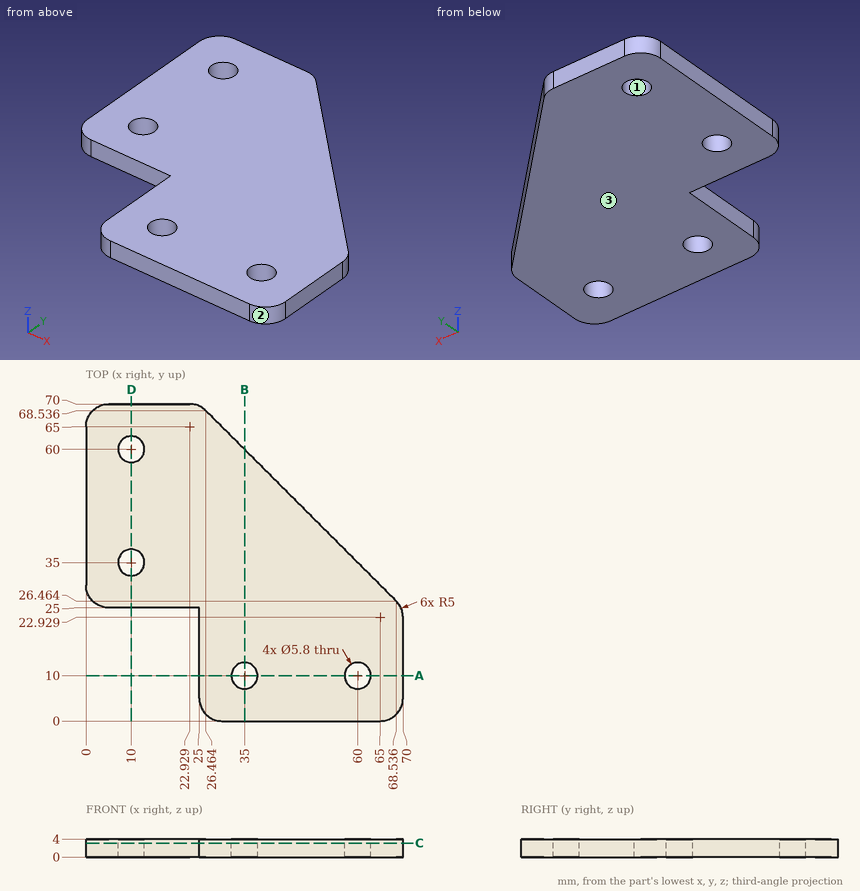
Answer from the drawing. Dimensions are ordinates in mm from the lowest x, y and z of the part. Give positions to 0.01 mm unless a question says otherwise; leave off trailing zeros. Loops run counter-clockwise (first coordinate to the right, second up) from the corner with the lowest first, then second, coordinate; pieces in that order, holes last. Notation, with made-up numbers: M -29.5,28.25 L 26.5,28.25 A7 ccw 26.5,36.25 Z; hole C 28,51.5 d7. An arc over 180 degrees is marked long. One line per item, written item: value.
Q1. Find the intervals of material crossed by line 1 (X direction, y = 10, z = 2.85); line 2 (X direction, y = 18, z = 2.45), in increasing order. Write a range as from..to.
Working result:
line 1: x = 25..32.1, 37.9..57.1, 62.9..70
line 2: x = 25..70
Q2. Determine the mould class of the marked faces 1, 2 and 3 for opening direction X: +X half, -X half, draft (parallel to the pull), parting line (faces both ways), or undercut.
Working result:
face 1: undercut
face 2: +X half
face 3: draft
Q3. A cutting plane is placed at B-B on x = 35. Determine the outline of the cut face in (y, z).
Working result:
outline: M 0,0 L 7.1,0 L 7.1,4 L 0,4 Z; M 12.9,0 L 60,0 L 60,4 L 12.9,4 Z
Q4. A cutting plane is placed at A-A on y = 10. Determine the outline of the cut face in (x, z), then the cut area to 3 significant figures.
Working result:
outline: M 25,0 L 32.1,0 L 32.1,4 L 25,4 Z; M 37.9,0 L 57.1,0 L 57.1,4 L 37.9,4 Z; M 62.9,0 L 70,0 L 70,4 L 62.9,4 Z
area: 134 mm^2
Q5. Flat-ended cylindrical pins translate along their axes: P1, Ø6.5, axis at x = 60, y = 10, coming from the +Z side; P2, Ø4.5, axis at x = 10, y = 35, coming from the -Z side; P3, Ø1.5, axis at y = 47.5, z = 1, coming from the +X side; P4, Ø1.2, axis at y = 10.5, z = 1.5, coming from the -X side. Find the tip coordinate at first contact, or state that the pin passes through.
Working result:
P1: stops at z = 4
P2: passes through
P3: stops at x = 48.25
P4: stops at x = 25
Q6. A cutting plane is placed at C-C on z = 3.1. Determine the outline of the cut face in (x, y) (1 decimal).
Working result:
outline: M 0,30 A5 ccw 5,25 L 25,25 L 25,5 A5 ccw 30,0 L 65,0 A5 ccw 70,5 L 70,22.9 A5 ccw 68.5,26.5 L 26.5,68.5 A5 ccw 22.9,70 L 5,70 A5 ccw 0,65 Z; hole C 10,35 d5.8; hole C 10,60 d5.8; hole C 35,10 d5.8; hole C 60,10 d5.8
